Geometry: see drawing. Coordinates: mm, zero at the bounding-box minimum. A direction names the side the tool comes from. Coordinates: 2 decimals unless noted, no trailing zeros. Order: outer loops, then holes, each group sorted by start corner. A loop starts at its lowest first (then second) coordinate and runs counter-clockwise, first axis right, second up. Notation, with made-up numbers: (-20.5, 6.25) -> (9.5, 6.25) arc R14 cw to (9.5, 25.25) -> close; hole circle Ø8 at (-28, 58.25). An arc over 180 degrees is marked (long way). Write each question's results on one line, items separated by ' | '.
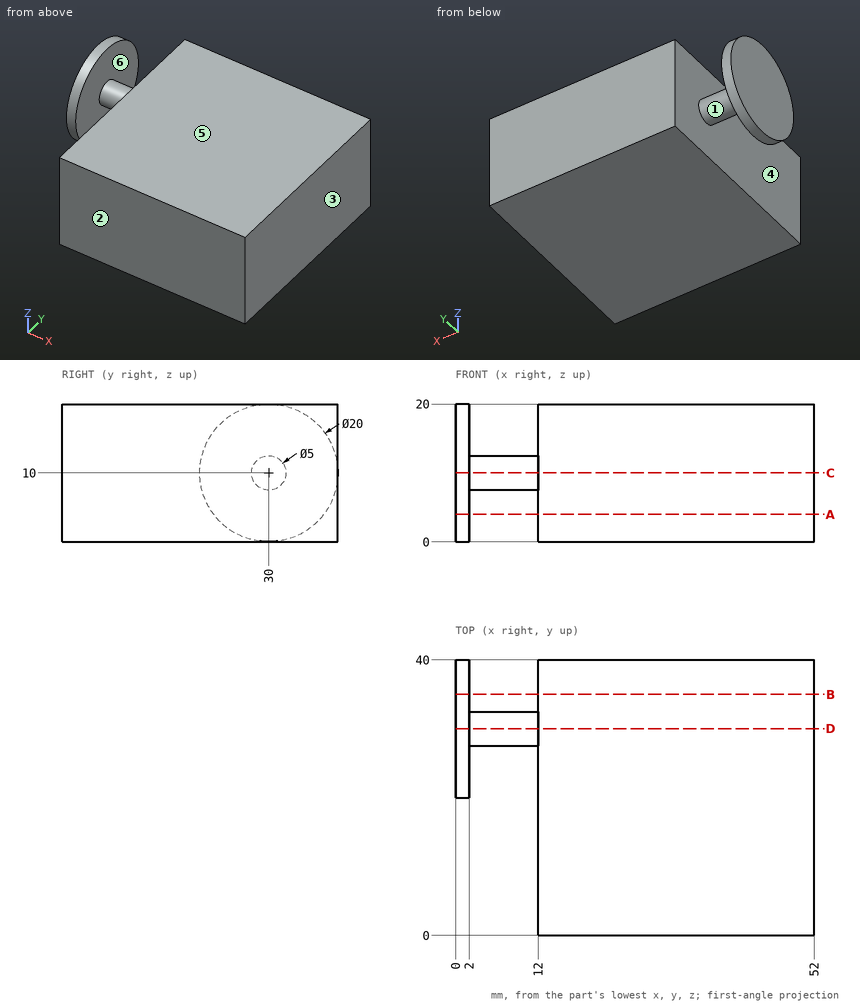
(1) Pin query (flat end, axial travel): P1, Ø10, axis at y = 14, z = 11, coming from the -X side. Return the tip coordinate at first contact, or that it passes through.
Return value:
P1: x = 12
(2) Reachability of the marked faces 1 and 2 from +Z, -Z, +X, -X, +Y, -Y: full face, straight path, thin tool, end or side. Return the list, or none.
Return value:
face 1: none | face 2: +Z, -Z, +X, -X, -Y
(3) Cut plane C-C, the plane z = 10. Return loops of the section in (x, y), plus the area to 3 significant figures.
Return value:
outline: (0, 20) -> (2, 20) -> (2, 27.5) -> (12, 27.5) -> (12, 0) -> (52, 0) -> (52, 40) -> (12, 40) -> (12, 32.5) -> (2, 32.5) -> (2, 40) -> (0, 40) -> close | area: 1,690 mm2
(4) Cut plane D-D, the plane y = 30. Return loops of the section in (x, z), plus the area to 3 significant figures.
Return value:
outline: (0, 0) -> (2, 0) -> (2, 7.5) -> (12, 7.5) -> (12, 0) -> (52, 0) -> (52, 20) -> (12, 20) -> (12, 12.5) -> (2, 12.5) -> (2, 20) -> (0, 20) -> close | area: 890 mm2
(5) Mould query, pull axis X, two halves, no side actions, for the marked faces 3, 4, 5 and 6. Classes: +X half, -X half, draft (parallel to the pull), parting line (faces both ways), or undercut.
Return value:
face 3: +X half | face 4: undercut | face 5: draft | face 6: undercut
(6) Cut plane B-B, the plane y = 35. Return loops of the section in (x, z), plus the area to 3 significant figures.
Return value:
outline: (0, 1.34) -> (2, 1.34) -> (2, 18.66) -> (0, 18.66) -> close; (12, 0) -> (52, 0) -> (52, 20) -> (12, 20) -> close | area: 835 mm2
(7) Cut plane A-A, the plane z = 4. Return loops of the section in (x, y), plus the area to 3 significant figures.
Return value:
outline: (0, 22) -> (2, 22) -> (2, 38) -> (0, 38) -> close; (12, 0) -> (52, 0) -> (52, 40) -> (12, 40) -> close | area: 1,630 mm2
(8) Line query: line 1 along X through (y, z) = (36.5, 12.25); line 2 along X through (y, z) = (10, 18.75); line 3 along Y through (x, z) = (11, 9.25). Output: solid intervals per line, ascending. Write a range as from..to.
Return value:
line 1: 0..2, 12..52 | line 2: 12..52 | line 3: 27.62..32.38
